from build123d import *

# Parameters (mm, degrees)
F0_W           = 80
F0_H           = 120
F1_DEPTH       = 15
F3_DEPTH       = 10
F5_D           = 4
F5_CSINK_D     = 8
F5_CSINK_ANGLE = 90


with BuildPart() as f1:
    # F0 (on Top) → F1 (new body)
    with BuildSketch(Plane.XY):
        Rectangle(F0_W, F0_H)
    extrude(amount=F1_DEPTH)

    # F2 (on face) → F3 (cut)
    with BuildSketch(Plane.XY.offset(15)):
        Polygon((-11.2589411438, 15), (-2.5, 15), (-2.5, -60), (0, -60), (2.5, -60), (2.5, 15), (11.2589411438, 15), (11.2589411438, 42), (-11.2589411438, 42), align=None)
    extrude(amount=-F3_DEPTH, mode=Mode.SUBTRACT)

    # F5 (through all)
    with Locations(Plane.XY.offset(15)):
        with Locations((-26.7064720392, 47.5818291306), (26.7064720392, 47.5818291306)):
            CounterSinkHole(F5_D / 2, F5_CSINK_D / 2, counter_sink_angle=F5_CSINK_ANGLE)


solid = f1.part
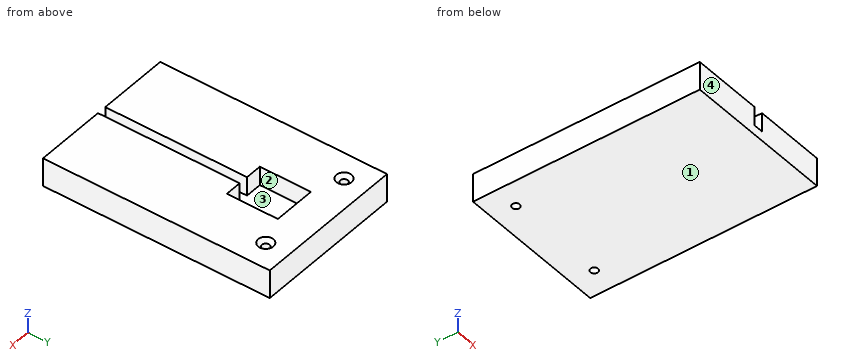
Source: CAD feature listing. Evaluate the final solid. Frame: model axes, mm. Face numbers are marked on the shaded views. Give positions to 0.01 mm unless a question says otherwise; leave off trailing zeros. Order: outer loops, then holes, each group sorted by start corner. A loop starts at its lowest first (then second) coordinate and runs counter-clockwise, first axis right, second up. Notation, with made-up numbers: (74, -35) -> (104, -35) arc R31 ccw to (104, -6) -> close; hole circle Ø10 at (11.25, -4). An arc over 180 degrees is marked (long way). Write item = value, one per line.
Q1. Material intervals for line 1 (X direction, y = 47.5, z = 8.75); line 2 (X direction, y = 0, z = 13.5); line 3 (X direction, y = 40, z = 7.75), sorted ascending. Write a range as from..to.
Data:
line_1 = -40..-28.7, -24.71..24.71, 28.7..40
line_2 = -40..-2.5, 2.5..40
line_3 = -40..-11.26, 11.26..40
Q2. Pin query (flat end, axial travel): pin 1 (3 mm diameter, centred on x = 26.71, y = 47.58, fed in from -Z). Return the tip coordinate at first contact, or that it passes through.
Data:
pin_1 = through
Q3. Cut plane B-B, the plane x = -9.5. Output: boundary loops of the cut face in (y, z).
Data:
outline = (-60, 0) -> (60, 0) -> (60, 15) -> (42, 15) -> (42, 5) -> (15, 5) -> (15, 15) -> (-60, 15) -> close
Q4. Pull-direction query (Y, two-part tool) for the marked faces 1, 2, 3 and 4; classes: released by +Y, released by -Y, zero draft, split by the parting line, or undercut.
Data:
face_1 = zero draft
face_2 = undercut
face_3 = undercut
face_4 = released by -Y
Q5. Cut plane C-C, the plane z = 11.75. Output: boundary loops of the cut face in (x, y).
Data:
outline = (-40, -60) -> (-2.5, -60) -> (-2.5, 15) -> (-11.26, 15) -> (-11.26, 42) -> (11.26, 42) -> (11.26, 15) -> (2.5, 15) -> (2.5, -60) -> (40, -60) -> (40, 60) -> (-40, 60) -> close; hole circle Ø4 at (-26.71, 47.58); hole circle Ø4 at (26.71, 47.58)
Q6. Cut plane A-A, the plane y = 4. Output: boundary loops of the cut face in (x, z).
Data:
outline = (-40, 0) -> (40, 0) -> (40, 15) -> (2.5, 15) -> (2.5, 5) -> (-2.5, 5) -> (-2.5, 15) -> (-40, 15) -> close
